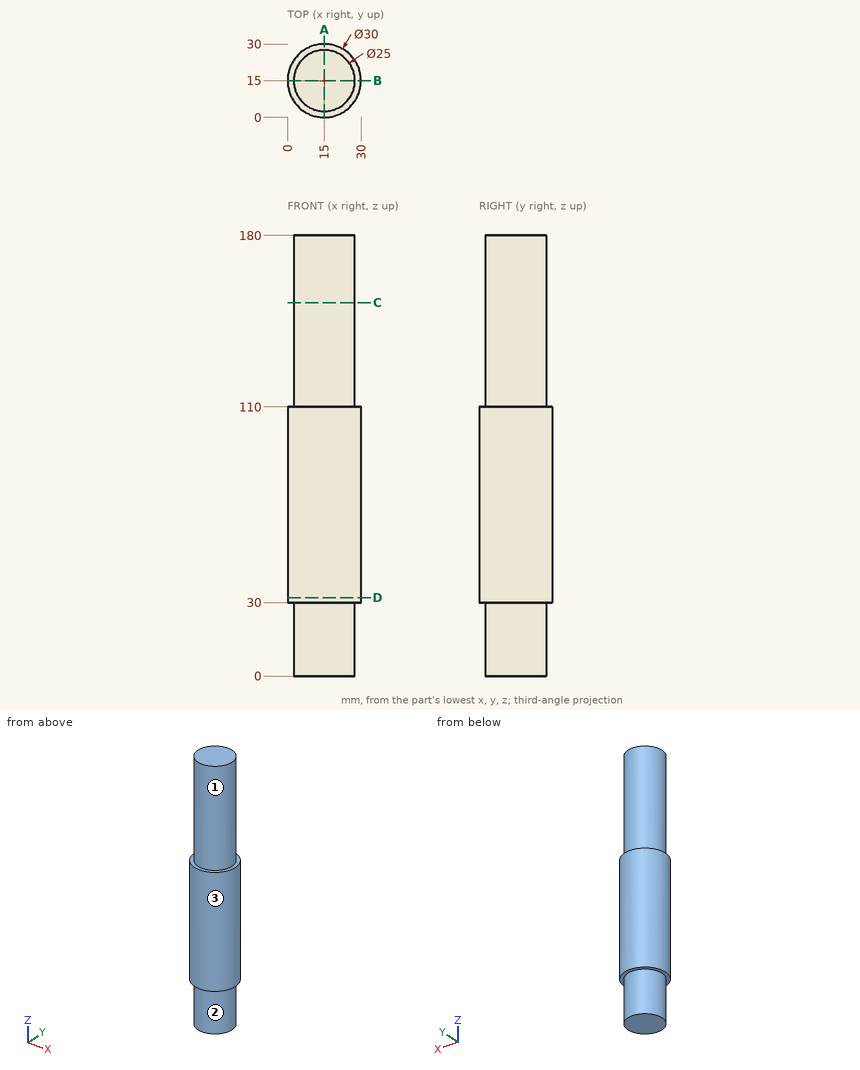
Geometry check sheet. Reference: drawing and pictorial views, mm from the part's lowest x, y, z. A direction names the side the tool comes from. Give positions to 0.01 mm unless a question says otherwise; leave off trailing zeros. Loops run counter-clockwise (first coordinate to the right, second up) from the corner with the lowest first, then second, coordinate; pieces in that order, holes last.
1. Section check C-C, the plane z = 152.5. Enter the section's corners in (x, y), then the cut area to 3 significant figures.
2. Go/stop test with flat-tipped pins: pin 1 Ø8 at (x, z) = (23.5, 157) entering from -Y; pin 2 Ø15 at (x, y) = (14.5, 13) entering from -Z; pin 3 Ø10 at (x, z) = (17.5, 144) entering from -Y; pin 4 Ø4 at (y, z) = (9.5, 122) entering from +X. Record where each tip stops, or that it passes through.
3. Thickness scan on line 1 (Z direction, x = 9.5, y = 28); line 2 (Y direction, x = 14.25, z = 159.5); line 3 (Y direction, x = 14.5, z = 93). Record the ranges inside material, lowest first.
4. Section check D-D, the plane z = 32. Enter the section's corners in (x, y), then the cut area to 3 significant figures.
5. Section check A-A, the plane x = 15. Enter the section's corners in (y, z).
6. Set-up check for the marked faces 1, 2 and 3: record each of +Z, -Z, +X, -X, +Y, -Y from which the full face is reachable in a straight line by a thin tool's end or side.
Geometry says:
1. outline: circle Ø25 at (15, 15)
1. area: 491 mm2
2. pin 1: stops at y = 3.34
2. pin 2: stops at z = 0
2. pin 3: stops at y = 2.5
2. pin 4: stops at x = 27
3. line 1: z = 30 to 110
3. line 2: y = 2.52 to 27.48
3. line 3: y = 0.01 to 29.99
4. outline: circle Ø30 at (15, 15)
4. area: 707 mm2
5. outline: (0, 30) - (2.5, 30) - (2.5, 0) - (27.5, 0) - (27.5, 30) - (30, 30) - (30, 110) - (27.5, 110) - (27.5, 180) - (2.5, 180) - (2.5, 110) - (0, 110) - close
6. face 1: +Z
6. face 2: -Z
6. face 3: +Z, -Z
